The model under review builds one solid part; all positions refer to its coordinate system, in mm. A direction names the side the tool comes from. Round coordinates to 2 decimals unless told otherwise and drop trailing zeros. Write each loop counter-clockwise with the first axis right and the second up, starting at its lowest first coordinate (ties: lowest second). Pieces come first, ordered by that corner, then holes. Notation, with made-up numbers: M 0,46 L 18,46 A15 cw 18,57 Z; hole C 27,89 d11. An arc over 180 degrees is marked long. Write item = value, one per line. Start each with the question number.
Item 1: The part is to be moulded in two halves that separate along Y. For faces 1 (the cylindrical face through (-20.506, -97.994, -78.88)), 2 (the cylindrical face through (-19.494, 183.494, -78.88)), 3 (the flat face through (-41, 43, 0)), 4 (the cylindrical face through (-25.825, 179.633, -78.88)), say which applies: +Y half, -Y half, draft (parallel to the pull), parting line (faces both ways), or undercut.
Item 2: To check wall thickness, follow line 1 along Z through (x, y) = (-2, -70); line 2 along Y through (x, z) = (-2.15, -140); line 3 along Y through (x, z) = (-2.1, -20). State the ranges of each line that lie inside material, in increasing order.
Item 3: Tool access review of faces 5 (the cylindrical face through (-41.52, 126.83, -31.5)), 6 (the flat face through (-3, -75, -81)), 7 (the flat face through (0, 155, -81)): name each direction out of +Z, -Z, +X, -X, +Y, -Y from which nothing blocks a thin tool from reaching the whole face with its end or side.
Item 4: Take a section at C-C, the plane y = 113. Give the boundary of the cut face in (x, z).
Item 5: For pin 1 Ø2.5 at (x, z) = (-1.5, -84.5) entering from -Y; pin 2 Ø1.5 at (x, z) = (-13.5, -140.5) entering from -Y; pin 3 Ø11 at (y, z) = (-69, -86.5) entering from +X, all flat-tipped, find the tip position at first contact; note any pin that passes through.
Item 6: Take a section at A-A, the plane x = -20. Give the boundary of the cut face in (y, z), plus the area to 3 significant figures.
Item 7: Take a section at B-B, the plane z = -109. Give the boundary of the cut face in (x, y), plus the area to 3 significant figures.
Item 8: Take a section at D-D, the plane z = -150. Give the boundary of the cut face in (x, y), plus the area to 3 significant figures.
from build123d import *

# Parameters (mm, degrees)
BOSS_EXTRUDE1_DEPTH = 160
SKETCH5_W           = 3
SKETCH5_H           = 21.357816692
BOSS_EXTRUDE4_DEPTH = 160
SKETCH7_R           = 1.5
CUT_EXTRUDE2_DEPTH  = 7
CUT_EXTRUDE3_DEPTH  = 3


with BuildPart() as part:
    # Sketch1 → Boss-Extrude1 (new body)
    with BuildSketch(Plane.XY):
        with BuildLine():
            Line((-40, -75), (-40, 160.5))
            ThreePointArc((-40, 160.5), (-20, 180.5), (0, 160.5))
            Line((0, 160.5), (3, 160.5))
            ThreePointArc((3, 160.5), (-20, 183.5), (-43, 160.5))
            Line((-43, 160.5), (-43, -75))
            ThreePointArc((-43, -75), (-20, -98), (3, -75))
            Line((3, -75), (0, -75))
            ThreePointArc((0, -75), (-20, -95), (-40, -75))
        make_face()
    extrude(amount=-BOSS_EXTRUDE1_DEPTH)

    # Sketch5 → Boss-Extrude4 (add)
    with BuildSketch(Plane(origin=(0, 0, -160), x_dir=(-1, 0, 0), z_dir=(0, 0, -1))):
        with Locations((1.5, -75.678908346)):
            Rectangle(SKETCH5_W, SKETCH5_H)
        with Locations((1.5, 161.178908346)):
            Rectangle(SKETCH5_W, SKETCH5_H)
    extrude(amount=-BOSS_EXTRUDE4_DEPTH)

    # Sketch7 → Cut-Extrude2 (cut, through all)
    with BuildSketch(Plane.ZY.offset(3)):
        with Locations((-140, -70)):
            Circle(SKETCH7_R)
        with Locations((-20, -70)):
            Circle(SKETCH7_R)
        with Locations((-20, 155.5)):
            Circle(SKETCH7_R)
        with Locations((-140, 155.5)):
            Circle(SKETCH7_R)
    extrude(amount=-CUT_EXTRUDE2_DEPTH, mode=Mode.SUBTRACT)

    # Sketch8 → Cut-Extrude3 (cut)
    with BuildSketch(Plane.ZY.offset(43)):
        with BuildLine():
            Line((-125, 128.257283518), (-35, 128.257283518))
            ThreePointArc((-35, 128.257283518), (-31.464466094, 126.792817424), (-30, 123.257283518))
            Line((-30, 123.257283518), (-30, 83.257283518))
            ThreePointArc((-30, 83.257283518), (-31.464466094, 79.721749612), (-35, 78.257283518))
            Line((-35, 78.257283518), (-125, 78.257283518))
            ThreePointArc((-125, 78.257283518), (-128.535533906, 79.721749612), (-130, 83.257283518))
            Line((-130, 83.257283518), (-130, 123.257283518))
            ThreePointArc((-130, 123.257283518), (-128.535533906, 126.792817424), (-125, 128.257283518))
        make_face()
    extrude(amount=-CUT_EXTRUDE3_DEPTH, mode=Mode.SUBTRACT)


solid = part.part
Response values:
q1.face_1 = -Y half
q1.face_2 = +Y half
q1.face_3 = draft
q1.face_4 = undercut
q2.line_1 = -160 to -141.5, -138.5 to -21.5, -18.5 to 0
q2.line_2 = -89.5 to -71.5, -68.5 to -65, 150.5 to 154, 157 to 175
q2.line_3 = -89.44 to -71.5, -68.5 to -65, 150.5 to 154, 157 to 174.94
q3.face_5 = +X, -X
q3.face_6 = +Z, -Z
q3.face_7 = +Z, -Z, +X
q4.outline = M -43,-160 L -40,-160 L -40,-130 L -43,-130 Z; M -43,-30 L -40,-30 L -40,0 L -43,0 Z
q5.pin_1 = -90.21
q5.pin_2 = -97.27
q5.pin_3 = 0
q6.outline = M -98,-160 L -95,-160 L -95,0 L -98,0 Z; M 180.5,-160 L 183.5,-160 L 183.5,0 L 180.5,0 Z
q6.area = 960 mm2
q7.outline = M -43,-75 A23 ccw 3,-75 L 0,-75 L 0,-65 L -3,-65 L -3,-85.54 A20 cw -40,-75 L -40,78.26 L -43,78.26 Z; M -43,128.26 L -40,128.26 L -40,160.5 A20 cw -3,171.04 L -3,150.5 L 0,150.5 L 0,160.5 L 3,160.5 A23 ccw -43,160.5 Z
q7.area = 1,060 mm2
q8.outline = M -43,-75 A23 ccw 3,-75 L 0,-75 L 0,-65 L -3,-65 L -3,-85.54 A20 cw -40,-75 L -40,160.5 A20 cw -3,171.04 L -3,150.5 L 0,150.5 L 0,160.5 L 3,160.5 A23 ccw -43,160.5 Z
q8.area = 1,210 mm2
